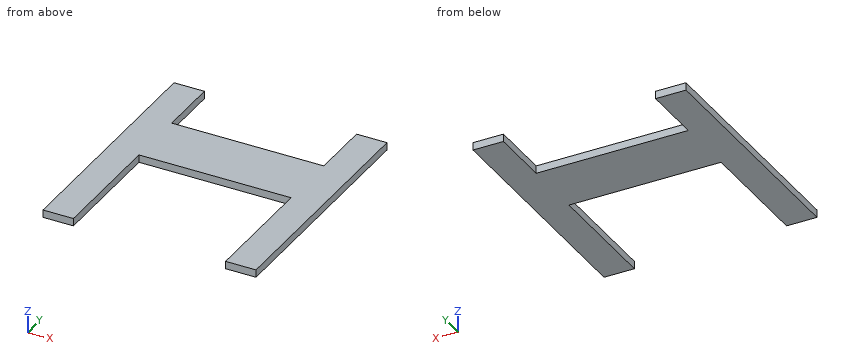
from build123d import *

# Parameters (mm, degrees)
F0_W     = 254
F0_H     = 101.6
F1_DEPTH = 12.7


with BuildPart() as f1:
    # F0 (on Top) → F1 (new body)
    with BuildSketch(Plane.XY):
        with Locations((0, 76.2)):
            Rectangle(F0_W, F0_H)
        Polygon((-177.8, 228.6), (-177.8, -177.8), (-127, -177.8), (-127, 25.4), (-127, 127), (-127, 228.6), align=None)
        Polygon((127, 127), (127, 25.4), (127, -177.8), (177.8, -177.8), (177.8, 228.6), (127, 228.6), align=None)
    extrude(amount=F1_DEPTH)


solid = f1.part
The model under review builds one solid part; all positions refer to its coordinate system, in mm. Coordinates: 2 decimals unless noted, no trailing zeros. Loops run counter-clockwise (first coordinate to the right, second up) from the corner with the lowest first, then second, coordinate; pieces in that order, holes last. Notation, with made-up numbers: (-5.5, -4.5) -> (23.5, -4.5) arc R14 cw to (23.5, 20.5) -> close; hole circle Ø5 at (11.25, 16.25). An arc over 180 degrees is marked (long way). Use a Markdown table: item, result. Add a question column.
1. Clearance check with flat-ended pins moving along their axes: pin 1 Ø2 at (x, z) = (125, 8) entering from -Y; pin 2 Ø4 at (x, z) = (-9.5, 6) entering from +Y. State where each tip first meets the part, or that it passes through.
2. Add section C-C on x = 102. Write out the cut boundary in (y, z), plus the area to 3 significant figures.
3. To check wall thickness, follow line 1 (X direction, y = -111.5, z = 10.5); line 2 (Y direction, x = -125, z = 6). State the ranges of each line that lie inside material, in increasing order.
4. Add section A-A on y = -14. Write out the cut boundary in (x, z).
5. Add section B-B on z = 10.75. Write out the cut boundary in (x, y), plus the area to 3 significant figures.
Returned:
| question | item | result |
|---|---|---|
| 1 | pin 1 | stops at y = 25.4 |
| 1 | pin 2 | stops at y = 127 |
| 2 | outline | (25.4, 0) -> (127, 0) -> (127, 12.7) -> (25.4, 12.7) -> close |
| 2 | area | 1,290 mm² |
| 3 | line 1 | x = -177.8 to -127, 127 to 177.8 |
| 3 | line 2 | y = 25.4 to 127 |
| 4 | outline | (-177.8, 0) -> (-127, 0) -> (-127, 12.7) -> (-177.8, 12.7) -> close; (127, 0) -> (177.8, 0) -> (177.8, 12.7) -> (127, 12.7) -> close |
| 5 | outline | (-177.8, -177.8) -> (-127, -177.8) -> (-127, 25.4) -> (127, 25.4) -> (127, -177.8) -> (177.8, -177.8) -> (177.8, 228.6) -> (127, 228.6) -> (127, 127) -> (-127, 127) -> (-127, 228.6) -> (-177.8, 228.6) -> close |
| 5 | area | 67,100 mm² |
